Autodesk Inventor part; units mm, degrees
ref_plane "YZ Plane" through (0, 0, 0) normal (1, 0, 0) x (0, 1, 0)
ref_plane "XZ Plane" through (0, 0, 0) normal (0, 1, 0) x (-1, 0, 0)
ref_plane "XY Plane" through (0, 0, 0) normal (0, 0, 1) x (1, 0, 0)
sketch "Sketch1" plane through (0, 0, 0) normal (1, 0, 0) x (0, 1, 0)
  line L0 (-70, 40) -> (50, 40)
  line L1 (90, 0) -> (90, 0)
  line L2 (50, -40) -> (-70, -40)
  line L3 (-90, -20) -> (-90, 20)
  line L4 (-90, 40) -> (90, -40) construction
  line L5 (90, 40) -> (-90, -40) construction
  circle A0 centre (55, 0) radius 11
  line L6 (0, 0) -> (0, -40.3764)
  circle A1 centre (-55, 0) radius 18
  arc A2 (90, 0) -> (50, 40) centre (50, 0) ccw
  arc A3 (50, -40) -> (90, 0) centre (50, 0) ccw
  arc A4 (-70, 40) -> (-90, 20) centre (-70, 20) ccw
  arc A5 (-90, -20) -> (-70, -40) centre (-70, -20) ccw
  dimension "d0" = 180
  dimension "d1" = 22
  dimension "d2" = 36
  dimension "d3" = 110
  dimension "d4" = 80
  dimension "d5" = 40
  dimension "d6" = 20
extrude "Extrusion1" add sketch "Sketch1" along normal mid plane 80
fillet "Fillet1" radius 10 12 edges at (40, -84.1421, 34.1421) (40, -90, 0) (40, -84.1421, -34.1421) (40, -10, -40) (40, 78.2843, 28.2843) (40, -10, 40) (-40, 78.2843, -28.2843) (-40, -10, -40) (-40, -84.1421, -34.1421) (-40, -90, 0) (-40, -84.1421, 34.1421) (-40, -10, 40)
sketch "Sketch2" plane through (-30, -70, 40) normal (0, 0, 1) x (1, 0, 0)
  line L0 (0, 160) -> (60, 160)
  line L1 (15, 160) -> (45, 160)
  line L2 (45, 160) -> (45, 100)
  line L3 (45, 100) -> (15, 100)
  line L4 (15, 100) -> (15, 160)
  line L5 (15, -20) -> (45, -20)
  line L6 (45, -20) -> (45, 50)
  line L7 (45, 50) -> (15, 50)
  line L8 (15, 50) -> (15, -20)
  line L9 (0, -20) -> (60, -20)
  line L10 (30, 160) -> (30, 100) construction
  point P0 (30, 70)
  dimension "d10" = 60
  dimension "d11" = 70
  dimension "d12" = 30
extrude "Extrusion2" cut sketch "Sketch2" against normal through all
fillet "Fillet2" radius 8 4 edges at (-15, 30, 0) (15, 30, 0) (-15, -20, 0) (15, -20, 0)
equation "\"d5\" = 0.5 * d4"
properties part number "Link_Tensionador"
Can you work these out from the model? Positions are in its coordinate system, mm. A direction names the side the tool comes from. Round coordinates to 2 decimals unless told otherwise and drop trailing zeros. Loops run counter-clockwise (first coordinate to the right, second up) from the corner with the lowest first, then second, coordinate; pieces in that order, holes last. Notation, with made-up numbers: (55, -32) - (113, -32) arc R32 cw to (113, 4) - close; hole circle Ø2 at (13, -24). An arc over 180 degrees is marked (long way). Answer in a Markdown table with one row per item. Add a question column.
Q1. I want a section at C-C on y = -22. List the corners of the cut face in (x, z) for me.
Q2. I want a section at B-B on x = -18. List the corners of the cut face in (y, z) for me.
Q3. We'd pull the mould along Z, two halves only. Please class faces 1 (the cylindrical face through (-27.325, -68.267, 12.165)), 2 (the cylindrical face through (37.15, -86.99, -0.28)), 3 (the cylindrical face through (22.395, -83.986, -34.297)): pulls with the +Z half, pulls with the -Z half, needs draft (parallel to the pull), parting line crosses it, or undercut.
Q4. For pin 1 Ø15.5 at (x, z) = (-2, 15.5) entering from +Y; pin 2 Ø4 at (x, z) = (0.5, 10) entering from -Y; pin 3 Ø4 at (x, z) = (-11.5, 19) entering from -Y, each with a flat end and sliding along its axis, tell me the tip position at first contact or that it passes through.
Q5. I want a section at A-A on y = -55. List the corners of the cut face in (x, z) for me, and give its area (3 significant figures).
Q6. Which directions (+Z, -Z, +X, -X, +Y, -Y) give clear straight access to the entire face, cutting with the end or side of a thin tool? Please do faces 4 (the cylindrical face through (-12.719, -22.406, -0.56)), 5 (the flat face through (0, 30, 1)), 6 (the cylindrical face through (-36.99, -9.16, -37.15)).
Q7. I want a section at D-D on z = 0. Count the separate pieces of the cut face and the enclosed holes in it, and give its area (3 significant figures).
Q8. I need wall thicknesses on L1, parallel to Y at x = 24, z = 0; L2, parallel to Z at x = 30.5, y = -55; L3, parallel to X at y = 50, z = -19.5. Which ranges of each line are inside material? Lowest first, please.
A:
| question | item | result |
|---|---|---|
| 1 | outline | (-40, -30) arc R10 ccw to (-30, -40) - (-12.29, -40) - (-12.29, 40) - (-30, 40) arc R10 ccw to (-40, 30) - close; (12.29, -40) - (30, -40) arc R10 ccw to (40, -30) - (40, 30) arc R10 ccw to (30, 40) - (12.29, 40) - close |
| 2 | outline | (-90, -20) arc R20 ccw to (-70, -40) - (50, -40) arc R40 ccw to (50, 40) - (-70, 40) arc R20 ccw to (-90, 20) - close; hole circle Ø36 at (-55, 0); hole circle Ø22 at (55, 0) |
| 3 | face 1 | undercut |
| 3 | face 2 | needs draft |
| 3 | face 3 | pulls with the -Z half |
| 4 | pin 1 | y = 30.49 |
| 4 | pin 2 | y = -20 |
| 4 | pin 3 | y = -23.34 |
| 5 | outline | (-40, -30) arc R10 ccw to (-30, -40) - (-15, -40) - (-15, -18) - (-40, -18) - close; (-40, 18) - (-15, 18) - (-15, 40) - (-30, 40) arc R10 ccw to (-40, 30) - close; (15, -40) - (30, -40) arc R10 ccw to (40, -30) - (40, -18) - (15, -18) - close; (15, 18) - (40, 18) - (40, 30) arc R10 ccw to (30, 40) - (15, 40) - close |
| 5 | area | 2,110 mm^2 |
| 6 | face 4 | +Z, -Z, -Y |
| 6 | face 5 | +Z, -Z, +Y |
| 6 | face 6 | -Z, -X, +Y, -Y |
| 7 | separate pieces | 5 |
| 7 | enclosed holes | 0 |
| 7 | area | 7,570 mm^2 |
| 8 | L1 | -90 to -73, -37 to 44, 66 to 90 |
| 8 | L2 | -39.99 to -18, 18 to 39.99 |
| 8 | L3 | -40 to -15, 15 to 40 |
